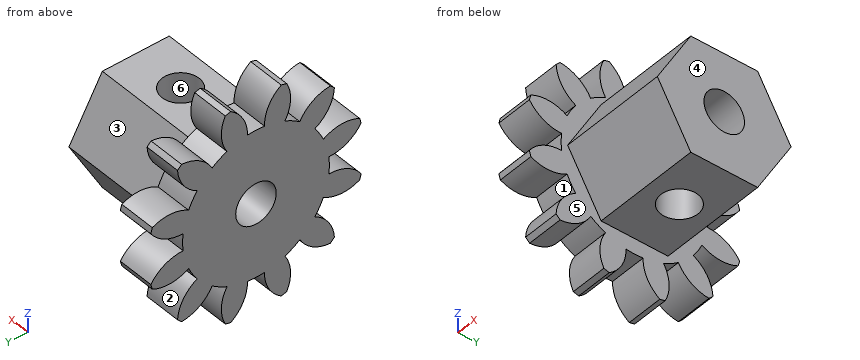
from build123d import *
from build123d.topology import SkipClean

# Parameters (mm, degrees)
BASPROSKE_W         = 4.7625
BASPROSKE_H         = 14
TOOTHCUT_DEPTH      = 21.36372771
TEETHCUTS_COUNT     = 12
TEETHCUTS_ANGLE     = 330
BORSKE_R            = 2.625
BORE_DEPTH          = 50.0000508
BOSS_EXTRUDE1_DEPTH = 13.99999994
SKETCH2_R           = 2.625
CUT_EXTRUDE1_DEPTH  = 27.882327142
SKETCH3_R           = 2.4
CUT_EXTRUDE2_DEPTH  = 32.354499992


with BuildPart() as part:
    # BasProSke → Base-Revolve (revolve)
    with BuildSketch(Plane(origin=(0, 0, 0), x_dir=(1, 0, 0), z_dir=(0, 1, 0)), mode=Mode.PRIVATE) as base_revolve_sk:
        with Locations((2.38125, 7)):
            Rectangle(BASPROSKE_W, BASPROSKE_H)
    revolve(base_revolve_sk.sketch.rotate(Axis((-10, 0, 0), (1, 0, 0)), 180), axis=Axis((-10, 0, 0), (1, 0, 0)))

    # TooCutSke → ToothCut (cut, through all)
    with BuildSketch(Plane(origin=(0, 0, 0), x_dir=(0, 0, -1), z_dir=(1, 0, 0))):
        with BuildLine():
            ThreePointArc((1.111908866, 9.433698091), (0, 9.499), (-1.111908866, 9.433698091))
            ThreePointArc((-1.111908866, 9.433698091), (-1.651516138, 11.821129337), (-3.298149691, 13.632096456))
            ThreePointArc((-3.298149691, 13.632096456), (0, 14.0254), (3.298149691, 13.632096456))
            ThreePointArc((3.298149691, 13.632096456), (1.651516138, 11.821129337), (1.111908866, 9.433698091))
        make_face()
    toothcut = extrude(amount=TOOTHCUT_DEPTH, mode=Mode.SUBTRACT)

    # TeethCuts: ToothCut ×12 about axis
    teethcuts_axis = Axis((-10, 0, 0), (1, 0, 0))
    for i in range(1, TEETHCUTS_COUNT):
        add(toothcut.rotate(teethcuts_axis, i * TEETHCUTS_ANGLE / (TEETHCUTS_COUNT - 1)), mode=Mode.SUBTRACT)

    # BorSke → Bore (cut, symmetric)
    with BuildSketch(Plane(origin=(0, 0, 0), x_dir=(0, 0, -1), z_dir=(1, 0, 0))):
        with Locations(Location((0, 0, 0), (0, 0, 180))):
            Circle(BORSKE_R)
    extrude(amount=BORE_DEPTH, both=True, mode=Mode.SUBTRACT)

    # Sketch1 → Boss-Extrude1 (add)
    with BuildSketch(Plane(origin=(4.7625, 0, 0), x_dir=(0, 0, -1), z_dir=(1, 0, 0))):
        Polygon((0, 8.660254038), (-7.5, 4.330127019), (-7.5, -4.330127019), (0, -8.660254038), (7.5, -4.330127019), (7.5, 4.330127019), align=None)
    extrude(amount=BOSS_EXTRUDE1_DEPTH)

    # Sketch2 → Cut-Extrude1 (cut, through all)
    with BuildSketch(Plane(origin=(18.76249994, 0, 0), x_dir=(0, 0, -1), z_dir=(1, 0, 0))):
        Circle(SKETCH2_R)
    extrude(amount=-CUT_EXTRUDE1_DEPTH, mode=Mode.SUBTRACT)

    # Sketch3 → Cut-Extrude2 (cut, through all)
    with SkipClean():  # the faces are left unmerged after this step: merging them gives an invalid solid
        with BuildSketch(Plane.XY.offset(7.5)):
            with Locations((11.76249997, 0)):
                Circle(SKETCH3_R)
        extrude(amount=-CUT_EXTRUDE2_DEPTH, mode=Mode.SUBTRACT)


solid = part.part
For this review, take the finished solid that the model builds, in its own axes (mm). Face numbers are marked on the shaded views. A direction names the side the tool comes from. Give positions to 0.01 mm unless a question says otherwise; leave off trailing zeros. Loops run counter-clockwise (first coordinate to the right, second up) from the corner with the lowest first, then second, coordinate; pieces in that order, holes last. Notation, with made-up numbers: M 50,-5 L 99,-5 A34 cw 99,31 Z; hole C 3.25,79 d2. An arc over 180 degrees is marked long. Put each result on its own line as item: value. Start each with the question number.
(1) For pin 1 (7 mm diameter, centred on x = 9, y = 0, fed in from +Z); pin 2 (3 mm diameter, centred on y = 10, z = 8, fed in from -X); pin 3 (6 mm diameter, centred on y = 9, z = -6.5, fed in from +X); pin 4 (7 mm diameter, centred on x = 13.5, y = 2, fed in from -Z), all flat-tipped, find the tip position at first contact; note any pin that passes through.
(2) Machinability: for the marked faces 5 and 6, which of the approach directions +Z, -Z, +X, -X, +Y, -Y give a long, thin tool a straight path to every point of the face, cutting with its end or side? Answer none if there is none.
(3) The part is to be moulded in two halves that separate along Z. For the marked faces 1, 2, 3 and 4, say which applies: +Z half, -Z half, draft (parallel to the pull), parting line (faces both ways), or undercut.
(4) Wall thickness on L1, parallel to Y at x = 14.5, z = 0 (3 decimals); L2, parallel to X at y = 0, z = -5; L3, parallel to Z at x = 7, y = 3.25: over which ranges is each line inside the solid? List them lowest first.
(5) Add section C-C, the plane z = -0.5. Write out the cut boundary in (x, y).
(6) Add section D-D, the plane z = -6.75. Write out the cut boundary in (x, y).
(7) Add section A-A, the plane y = 0. Write out the cut boundary in (x, z) (1 decimal).
(8) Add section B-B, the plane x = 8.5. Write out the cut boundary in (y, z) (3 decimals), then the cut area to 3 significant figures.
Result:
1. pin 1: stops at z = 7.5
1. pin 2: stops at x = 0
1. pin 3: stops at x = 4.76
1. pin 4: stops at z = -7.5
2. face 5: +X
2. face 6: +Z, -Z
3. face 1: undercut
3. face 2: undercut
3. face 3: +Z half
3. face 4: draft
4. L1: y = -8.66 to -2.625, 2.625 to 8.66
4. L2: x = 0 to 9.36, 14.16 to 18.76
4. L3: z = -7.5 to 7.5
5. outline: M 0,-9.49 L 4.76,-9.49 L 4.76,-8.37 L 18.76,-8.37 L 18.76,-2.58 L 0,-2.58 Z; M 0,2.58 L 18.76,2.58 L 18.76,8.37 L 4.76,8.37 L 4.76,9.49 L 0,9.49 Z
6. outline: M 0,-8.97 L 4.76,-8.97 L 4.76,-4.76 L 18.76,-4.76 L 18.76,4.76 L 4.76,4.76 L 4.76,8.97 L 0,8.97 Z; hole C 11.76,0 d4.8
7. outline: M 0,-9.5 L 4.8,-9.5 L 4.8,-7.5 L 9.4,-7.5 L 9.4,-2.6 L 0,-2.6 Z; M 0,2.6 L 9.4,2.6 L 9.4,7.5 L 4.8,7.5 L 4.8,9.5 L 0,9.5 Z; M 14.2,-7.5 L 18.8,-7.5 L 18.8,-2.6 L 14.2,-2.6 Z; M 14.2,2.6 L 18.8,2.6 L 18.8,7.5 L 14.2,7.5 Z
8. outline: M -8.66,0 L -4.33,-7.5 L 4.33,-7.5 L 8.66,0 L 4.33,7.5 L -4.33,7.5 Z; hole C 0,0 d5.25
8. area: 173 mm^2
